Autodesk Inventor part; units mm, degrees
ref_plane "YZ Plane" through (0, 0, 0) normal (1, 0, 0) x (0, 1, 0)
ref_plane "XZ Plane" through (0, 0, 0) normal (0, 1, 0) x (-1, 0, 0)
ref_plane "XY Plane" through (0, 0, 0) normal (0, 0, 1) x (1, 0, 0)
sketch "Sketch1" plane through (0, 0, 0) normal (0, 0, 1) x (1, 0, 0)
  line L0 (-11, 0) -> (-14, 0)
  line L1 (-14, 0) -> (-14, 10)
  line L2 (-14, 10) -> (-18, 10)
  line L3 (-18, 10) -> (-18, 12)
  line L4 (-18, 12) -> (-11, 12)
  line L5 (-11, 10) -> (-11, 0)
  line L6 (-11, 10) -> (-11, 12)
  line L7 (-6, 0) -> (-6, 10)
  dimension "d1" = 10
  dimension "d2" = 4
  dimension "d3" = 2
  dimension "d4" = 3
  dimension "d6" = 5
revolve "Revolution1" add sketch "Sketch1" angle 360 about axis through (-6, 0, 0) along (0, 1, 0)
properties part number "Buje para Tornillo" material "Brass, Soft Yellow"
Geometry: final body of the model. Coordinates: model frame, mm. A direction names the side the tool comes from. Round coordinates to 2 decimals unless told otherwise and drop trailing zeros. Loops run counter-clockwise (first coordinate to the right, second up) from the corner with the lowest first, then second, coordinate; pieces in that order, holes last. Notation, with made-up numbers: M 44,-29.75 L 75,-29.75 A16 ccw 75,-1.75 Z; hole C 46,41 d4. An arc over 180 degrees is marked long. Put each result on its own line as item: value. Start each with the question number.
(1) Material intervals for line 1 along Z through (x, y) = (-6, 7); line 2 along X through (y, z) = (10.5, -0.25); line 3 along X through (y, z) = (6.5, 1.25), sorted ascending. Write a range as [from, to].
(2) Section query A-A (x = -6). Return loops of the section in (y, z), then the cut area to 3 significant figures.
(3) Section query D-D (z = -7.5). Return loops of the section in (x, y).
(4) Contact query for flat-ended pins moving along their axis: pin 1 Ø1 at (x, y) = (-8.5, 2) entering from +Z; pin 2 Ø6 at (x, y) = (-14, 3) entering from +Z (3 decimals). Output: stop coordinate, or through.
(5) Draft query along X for faces 1 (the face through (-11.2, 12, 0.2)), 2 (the face through (-2, 6, -3)), 3 (the face through (-17.085, 11.014, -4.596)). Return one class per face: +X half, -X half, draft (parallel to the pull), parting line (faces both ways), or undercut.
(6) Section query B-B (z = 0). Return loops of the section in (x, y), then the cut area to 3 significant figures.
(7) Set-up query: faces 4 (the face through (-9.69, 5.07, -7.1)), 5 (the face through (-11.2, 0, 0.1)). Return all of +Z, -Z, +X, -X, +Y, -Y with unobstructed straight access to the full face (end or side cutting, diameter ignored); none if empty.
(8) Section query C-C (y = 3.75). Return loops of the section in (x, z), then the cut area to 3 significant figures.
Findings below:
1. line 1: z = [-8, -5], [5, 8]
1. line 2: x = [-18, -10.99], [-1.01, 6]
1. line 3: x = [-13.9, -10.84], [-1.16, 1.9]
2. outline: M 0,-8 L 10,-8 L 10,-12 L 12,-12 L 12,-5 L 0,-5 Z; M 0,5 L 12,5 L 12,12 L 10,12 L 10,8 L 0,8 Z
2. area: 88.0 mm2
3. outline: M -15.37,10 L -8.78,10 L -8.78,0 L -3.22,0 L -3.22,10 L 3.37,10 L 3.37,12 L -15.37,12 Z
4. pin 1: stops at z = 7.75
4. pin 2: stops at z = 6.245
5. face 1: draft
5. face 2: undercut
5. face 3: parting line
6. outline: M -18,10 L -14,10 L -14,0 L -11,0 L -11,12 L -18,12 Z; M -1,0 L 2,0 L 2,10 L 6,10 L 6,12 L -1,12 Z
6. area: 88.0 mm2
7. face 4: -Y
7. face 5: +Z, -Z, +X, -X, -Y
8. outline: C -6,0 d16; hole C -6,0 d10
8. area: 123 mm2
